Autodesk Inventor part; units mm, degrees
ref_plane "YZ Plane" through (0, 0, 0) normal (1, 0, 0) x (0, 1, 0)
ref_plane "XZ Plane" through (0, 0, 0) normal (0, 1, 0) x (-1, 0, 0)
ref_plane "XY Plane" through (0, 0, 0) normal (0, 0, 1) x (1, 0, 0)
sketch "Sketch1" plane through (0, 0, 0) normal (0, 1, 0) x (-1, 0, 0)
  circle A0 centre (0, 0) radius 23
  dimension "d0" = 46
extrude "Extrusion1" add sketch "Sketch1" along normal blind 7
sketch "Sketch2" plane through (0, 7, 0) normal (0, 1, 0) x (1, 0, 0)
  line L0 (-8.5, -35.5) -> (8.5, -35.5)
  line L1 (-8.5, -35.5) -> (-15, -17.4356)
  circle A0 centre (0, 0) radius 23
  line L2 (8.5, -35.5) -> (15, -17.4356)
  circle A1 centre (0, -28) radius 3.5
  point P0 (0, -35.5)
  dimension "d3" = 17
  dimension "d4" = 35.5
  dimension "d5" = 7
  dimension "d6" = 28
  dimension "d7" = 30
extrude "Extrusion2" add sketch "Sketch2" against normal blind 7 contours L1 A0 L2 L0
fillet "Fillet1" radius 5 2 edges at (15, 3.5, 17.4356) (-15, 3.5, 17.4356)
mirror "Mirror1" about plane through (0, 0, 0) normal (0, 0, 1) of "Extrusion2", "Fillet1"
sketch "Sketch3" plane through (0, 7, 0) normal (0, 1, 0) x (1, 0, 0)
  circle A0 centre (0, 0) radius 22
  dimension "d11" = 44
extrude "Extrusion3" add sketch "Sketch3" along normal blind 7
sketch "Sketch4" plane through (0, 14, 0) normal (0, 1, 0) x (1, 0, 0)
  circle A0 centre (0, 0) radius 11.5
  dimension "d14" = 23
extrude "Extrusion4" add sketch "Sketch4" along normal blind 5.5
sketch "Sketch5" plane through (0, 19.5, 0) normal (0, 1, 0) x (1, 0, 0)
  circle A0 centre (0, 0) radius 8.5
  dimension "d17" = 17
extrude "Extrusion5" cut sketch "Sketch5" against normal through all
sketch "Sketch6" plane through (0, 14, 0) normal (0, 1, 0) x (1, 0, 0)
  circle A0 centre (0, 0) radius 20
  circle A1 centre (0, 0) radius 11.5
  dimension "d20" = 40
extrude "Extrusion6" cut sketch "Sketch6" against normal blind 3
properties part number "HCMUTE-CDT23-GOI_DO_PHI-17" material "Stainless Steel"
Build history of the part. All positions in model axes, mm. A direction names the side the tool comes from. Coordinates: 2 decimals unless noted, no trailing zeros. Order: outer loops, then holes, each group sorted by start corner. A loop starts at its lowest first (then second) coordinate and runs counter-clockwise, first axis right, second up. Notation, with made-up numbers: (-38.75, -9) -> (-13.75, -9) arc R13 cw to (-13.75, 5) -> close; hole circle Ø6 at (46, 16.25). An arc over 180 degrees is marked (long way). Answer in a Markdown table with one row per item. Add a question column.
Q1. Band-saw the part on B-B, the plane x = 0. List the corners of the cut face in (y, z).
Q2. Wall check: line 1 along Z through (x, y) = (0, 6.5); line 2 along X through (y, z) = (13.25, 0). Give the ranges that are in metal, low to high. Write a range as [from, to].
Q3. Which spindle directions (+Z, -Z, +X, -X, +Y, -Y) get a long thin tool onto all of the face, cutting with end or side? Do faces 4 (the face through (-11.58, 3.55, -26.94)), 5 (the face through (10, 14, 18)). Say none if no direction does.
Q4. Band-saw the part on D-D, the plane x = -6.5. List the corners of the cut face in (y, z), then the cut area to 3 significant figures.
Q5. Band-saw the part on C-C, the plane y = 12.75. List the corners of the cut face in (x, z), then the cut area to 3 significant figures.
Q6. Band-saw the part on A-A, the plane z = 0. List the corners of the cut face in (x, y), then the cut area to 3 significant figures.
Q7. Mould opens along X. For faces 1 (the face through (-11.496, 3.549, 27.173)), 2 (the face through (-4.336, 12.521, 19.524)), 3 (the face through (-6.7, 7, 21.2)) say: +X half, -X half, draft (parallel to the pull), parting line (faces both ways), or undercut.
Q8. Drop flat-ended pins along their axis: pin 1 (8 mm diameter, centred on y = 3.5, z = 23, fed in from +X); pin 2 (10 mm diameter, centred on x = -10, y = 13, fed in from +Z); pin 3 (8 mm diameter, centred on x = 0, y = 14, fed in from -Z). Give the stop position or say it passes through.
Answers follow:
| question | item | result |
|---|---|---|
| 1 | outline | (0, -35.5) -> (7, -35.5) -> (7, -31.5) -> (0, -31.5) -> close; (0, -24.5) -> (7, -24.5) -> (7, -22) -> (14, -22) -> (14, -20) -> (11, -20) -> (11, -11.5) -> (19.5, -11.5) -> (19.5, -8.5) -> (0, -8.5) -> close; (0, 8.5) -> (19.5, 8.5) -> (19.5, 11.5) -> (11, 11.5) -> (11, 20) -> (14, 20) -> (14, 22) -> (7, 22) -> (7, 24.5) -> (0, 24.5) -> close; (0, 31.5) -> (7, 31.5) -> (7, 35.5) -> (0, 35.5) -> close |
| 2 | line 1 | [-35.5, -31.5], [-24.5, -8.5], [8.5, 24.5], [31.5, 35.5] |
| 2 | line 2 | [-22, -20], [-11.5, -8.5], [8.5, 11.5], [20, 22] |
| 3 | face 4 | -Z, -X, +Y, -Y |
| 3 | face 5 | +Y |
| 4 | outline | (0, -35.5) -> (7, -35.5) -> (7, -21.02) -> (14, -21.02) -> (14, -18.91) -> (11, -18.91) -> (11, -9.49) -> (19.5, -9.49) -> (19.5, -5.48) -> (0, -5.48) -> close; (0, 5.48) -> (19.5, 5.48) -> (19.5, 9.49) -> (11, 9.49) -> (11, 18.91) -> (14, 18.91) -> (14, 21.02) -> (7, 21.02) -> (7, 35.5) -> (0, 35.5) -> close |
| 4 | area | 625 mm^2 |
| 5 | outline | circle Ø44 at (0, 0); circle Ø23 at (0, 0); hole circle Ø40 at (0, 0); hole circle Ø17 at (0, 0) |
| 5 | area | 452 mm^2 |
| 6 | outline | (-23, 0) -> (-8.5, 0) -> (-8.5, 19.5) -> (-11.5, 19.5) -> (-11.5, 11) -> (-20, 11) -> (-20, 14) -> (-22, 14) -> (-22, 7) -> (-23, 7) -> close; (8.5, 0) -> (23, 0) -> (23, 7) -> (22, 7) -> (22, 14) -> (20, 14) -> (20, 11) -> (11.5, 11) -> (11.5, 19.5) -> (8.5, 19.5) -> close |
| 6 | area | 374 mm^2 |
| 7 | face 1 | -X half |
| 7 | face 2 | undercut |
| 7 | face 3 | draft |
| 8 | pin 1 | x = 14.44 |
| 8 | pin 2 | z = 21.42 |
| 8 | pin 3 | z = -22 |
